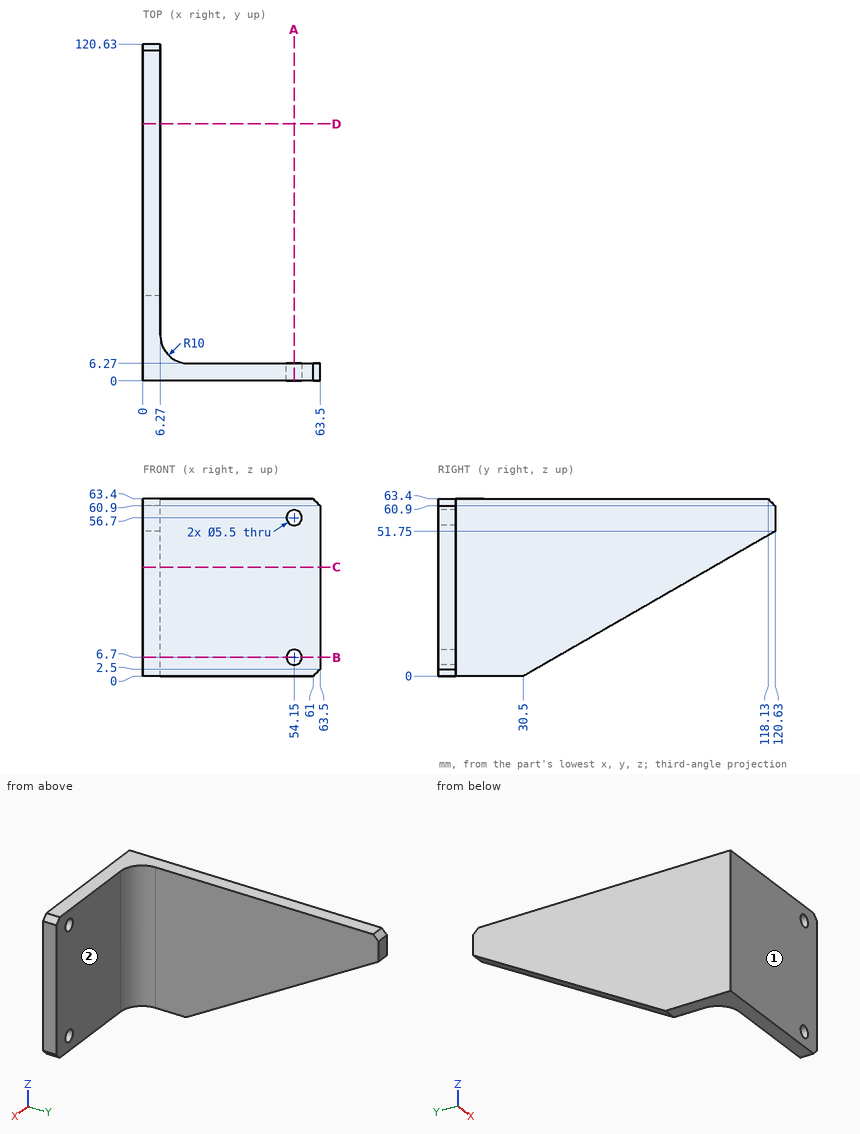
Design review of the part shown in the three views and the two pictorial views. Dimensions are in mm from the part's minimum x, y and z. A direction names the side the tool comes from. Give positions to 0.01 mm unless a question says otherwise; leave off trailing zeros. Write each loop counter-clockwise with the first axis right and the second up, starting at its lowest first coordinate (ties: lowest second). Pieces come first, ordered by that corner, then holes. Notation, with made-up numbers: M 53,80.25 L 87,80.25 A37 ccw 87,116.25 Z; hole C 64.25,53.5 d2. An arc over 180 degrees is marked long. Answer as CSV lines item,"result".
1. Wall thickness on line 1 (Z direction, x = 54.15, y = 3); line 2 (X direction, y = 4.25, z = 56.7); line 3 (Y direction, x = 36, z = 51): over which ranges is each line inside the solid? List them lowest first.
Findings:
line 1,"z = 0 to 3.95, 9.45 to 53.95, 59.45 to 63.4"
line 2,"x = 0 to 51.4, 56.9 to 63.5"
line 3,"y = 0 to 6.27"
2. Consider section A-A, the plane x = 54.15. Write out the cut boundary in (y, z).
Findings:
outline,"M 0,0 L 6.27,0 L 6.27,3.95 L 0,3.95 Z; M 0,9.45 L 6.27,9.45 L 6.27,53.95 L 0,53.95 Z; M 0,59.45 L 6.27,59.45 L 6.27,63.4 L 0,63.4 Z"
3. Consider section C-C, the plane z = 39. Write out the cut boundary in (x, y), then the cut area to 3 significant figures.
Findings:
outline,"M 0,0 L 63.5,0 L 63.5,6.27 L 16.27,6.27 A10 cw 6.27,16.27 L 6.27,98.42 L 0,98.42 Z"
area,"997 mm2"
4. For the marked faces 1 and 2, list the 3-axis set-ups (+Z, -Z, +X, -X, +Y, -Y) from which the entire face can be reached by the end or side of a thin tool; tool diameter is ignored.
Findings:
face 1,"+Z, -Z, +X, -X, -Y"
face 2,"+Z, -Z, +X, +Y"
5. For pin 1 (14 mm diameter, centred on x = 30, z = 40, fed in from +Y); pin 2 (8 mm diameter, centred on y = 13, z = 21, fed in from +X); pin 3 (4.5 mm diameter, centred on x = 54.15, z = 56.7, fed in from +Y), all flat-tipped, find the tip position at first contact; note any pin that passes through.
Findings:
pin 1,"stops at y = 6.27"
pin 2,"stops at x = 9.4"
pin 3,"passes through"
6. Consider section B-B, the plane z = 6.7. Write out the cut boundary in (x, y), then the cut area to 3 significant figures.
Findings:
outline,"M 0,0 L 51.4,0 L 51.4,6.27 L 16.27,6.27 A10 cw 6.27,16.27 L 6.27,42.17 L 0,42.17 Z; M 56.9,0 L 63.5,0 L 63.5,6.27 L 56.9,6.27 Z"
area,"610 mm2"
7. Consider section D-D, the plane y = 92. Write out the cut boundary in (x, z), then the cut area to 3 significant figures.
Findings:
outline,"M 0,35.31 L 6.27,35.31 L 6.27,63.4 L 0,63.4 Z"
area,"176 mm2"
